Part model, mm, in its own coordinate system. A direction names the side the tool comes from. Round coordinates to 2 decimals unless told otherwise and drop trailing zeros. Loops run counter-clockwise (first coordinate to the right, second up) from the corner with the lowest first, then second, coordinate; pieces in that order, holes last.
(1) Cut at B-B on z = 2. Count the separate pieces of the cut face and the enclosed holes in it, then the cut area to 3 significant figures.
(2) Tool access for faces 5 (the face through (3.44, 2.08, -0.04)), 6 (the face through (8.029, 5.948, 1.993)): list every direction of +Z, -Z, +X, -X, +Y, -Y with a clear straight run to the whole face (end or side of a thin tool).
(3) Cut at A-A on x = 6.25. List the corners of the cut face in (y, z).
(4) Probe probe 1 along Z at (x, y) = (21.75, 32.5); probe 2 along X at (y, z) = (17.5, 1); probe 3 along Y at (x, z) = (14.5, 1.35). List the from-to ranges inside material, lowest first.
(5) Mould opens along Y. For faces 1 (the face through (20, 39, -2.5)), 2 (the face through (8.111, 5.845, -1.993)), 3 (the face through (3.986, 3.938, -0.035)), 4 (the face through (21.571, 37.776, -0.035)) say: +Y half, -Y half, draft (parallel to the pull), parting line (faces both ways), or undercut.
(6) Flat gauge pins, fed straight in: pin 1 (1.5 mm diameter, centred on x = 20.5, y = 18.5, fed in from -Z); pin 2 (6.5 mm diameter, centred on x = 11, y = 26.5, fed in from +Z); pin 3 (1 mm diameter, centred on y = 34.5, z = 0.5, fed in from -X); pin 4 (3 mm diameter, centred on y = 6, z = 1.5, fed in from -X). Where does each tip first touch, or does it go through?
Autodesk Inventor part; units mm, degrees
ref_plane "YZ Plane" through (0, 0, 0) normal (1, 0, 0) x (0, 1, 0)
ref_plane "XZ Plane" through (0, 0, 0) normal (0, 1, 0) x (-1, 0, 0)
ref_plane "XY Plane" through (0, 0, 0) normal (0, 0, 1) x (1, 0, 0)
sketch "Sketch2" plane through (0, 0, 0) normal (0, 0, 1) x (1, 0, 0)
  circle A0 centre (21.7341, 39.015) radius 1.25
  arc A1 (5.7341, 4.015) -> (21.7341, 39.015) centre (-21.2393, 37.5029) ccw construction
  arc A2 (7.6159, 1.6787) -> (24.7322, 39.1205) centre (-21.2393, 37.5029) ccw
  arc A3 (3.8522, 6.3514) -> (18.7359, 38.9095) centre (-21.2393, 37.5029) ccw
  arc A4 (3.8522, 6.3514) -> (7.6159, 1.6787) centre (5.7341, 4.015) ccw
  arc A5 (24.7322, 39.1205) -> (18.7359, 38.9095) centre (21.7341, 39.015) ccw
  circle A6 centre (5.7341, 4.015) radius 1.75
  dimension "d18" = 6
  dimension "d21" = 40
  dimension "d22" = 35
  dimension "d23" = 16
  dimension "d24" = 2.5
  dimension "d26" = 3.5
extrude "Extrusion1" add sketch "Sketch2" along normal mid plane 3
sketch "Sketch3" plane through (0, 0, 1.5) normal (0, 0, 1) x (1, 0, 0)
  arc A0 (3.8522, 6.3514) -> (7.6159, 1.6787) centre (5.7341, 4.015) ccw
  arc A1 (24.7322, 39.1205) -> (18.7359, 38.9095) centre (21.7341, 39.015) ccw
  circle A2 centre (5.7341, 4.015) radius 1.75
  circle A3 centre (21.7341, 39.015) radius 1.25
  circle A4 centre (5.7341, 4.015) radius 3
  circle A5 centre (21.7341, 39.015) radius 3
  point P0 (0, 0)
  point P1 (18.7359, 38.9095)
  point P2 (24.7322, 39.1205)
  point P3 (7.6159, 1.6787)
  point P4 (3.8522, 6.3514)
extrude "Extrusion2" add sketch "Sketch3" along normal blind 1
mirror "Mirror1" about plane through (0, 0, 0) normal (0, 0, 1) of "Extrusion2"
properties part number "tolo"
Final values:
1. separate pieces: 2
1. enclosed holes: 2
1. area: 42.0 mm2
2. face 5: +Z, -Z
2. face 6: +Z
3. outline: (1.06, -2.5) - (2.34, -2.5) - (2.34, 2.5) - (1.06, 2.5) - close; (5.69, -2.5) - (6.97, -2.5) - (6.97, -1.5) - (8.45, -1.5) - (8.45, 1.5) - (6.97, 1.5) - (6.97, 2.5) - (5.69, 2.5) - close
4. probe 1: z = -1.5 to 1.5
4. probe 2: x = 13.4 to 20.18
4. probe 3: y = 8.54 to 19.54
5. face 1: draft
5. face 2: parting line
5. face 3: undercut
5. face 4: undercut
6. pin 1: stops at z = -1.5
6. pin 2: passes through
6. pin 3: stops at x = 18.61
6. pin 4: stops at x = 2.77
